Read the model definition and answer for the solid it produces. Units are mm, in the model's axes. Give positions to 0.01 mm unless a question says otherwise; leave off trailing zeros. Order: outer loops, then holes, each group sorted by start corner. A loop starts at its lowest first (then second) coordinate and runs counter-clockwise, first axis right, second up. Notation, with made-up numbers: (28.5, 83.25) - (64.5, 83.25) arc R5 cw to (64.5, 88.25) - close; hole circle Ø2 at (37.5, -38). An arc over 180 degrees is marked (long way). Return JSON: item names as keys, results as strings.
```python
from build123d import *

# Parameters (mm, degrees)
F0_R          = 11
F1_DEPTH      = 37
F3_DEPTH      = 11.001
F3_DEPTH_BACK = 11.001


with BuildPart() as f1:
    # F0 (on Top) → F1 (new body)
    with BuildSketch(Plane.XY):
        Circle(F0_R)
    extrude(amount=F1_DEPTH)

    # F2 (on Front) → F3 (cut, two sides)
    with BuildSketch(Plane.XZ) as f3_sk:
        Polygon((11, 37), (-11, 37), (-11, 34.5), align=None)
    extrude(amount=-F3_DEPTH, mode=Mode.SUBTRACT)
    extrude(f3_sk.sketch, amount=F3_DEPTH_BACK, mode=Mode.SUBTRACT)

    # F4 (on face) → F5 (revolve, cut)
    with BuildSketch(Plane(origin=(-4.010708822, 0, 35.2942376339), x_dir=(0.9936052548, 0, 0.112909688), z_dir=(-0.112909688, 0, 0.9936052548))):
        with BuildLine():
            Line((12.7865213476, 0), (-4.7134786524, 0))
            ThreePointArc((-4.7134786524, 0), (4.0365213476, -8.75), (12.7865213476, 0))
        make_face()
    revolve(axis=Axis((0, 0, 35.75), (0.9936052548, 0, 0.112909688)), mode=Mode.SUBTRACT)


solid = f1.part
```
Q1. A cutting plane is placed at B-B (z = 6). Write down the section's boundary in (x, y).
Values:
{"outline": "circle Ø22 at (0, 0)"}
Q2. Given pin 1 (12 mm diameter, centred on x = -7, z = 10.5, fed in from -Y); pin 2 (1 mm diameter, centred on x = 2, z = 19, fed in from -Y); pin 3 (4 mm diameter, centred on x = 3.5, z = 7.5, fed in from +Y), each flat-ended and moving along its own axis, determine where each tip first touches the part or whether it passes through.
Values:
{"pin 1": "stops at y = -10.95", "pin 2": "stops at y = -10.9", "pin 3": "stops at y = 10.9"}
Q3. A cutting plane is placed at D-D (z = 30). Write down the section's boundary in (x, y), and give its area (3 significant figures).
Values:
{"outline": "circle Ø22 at (0, 0); hole circle Ø13.19 at (0, 0)", "area": "243 mm²"}
Q4. A cutting plane is placed at A-A (x = 6.5). Write down the section's boundary in (y, z), and give its area (3 significant figures).
Values:
{"outline": "(-8.87, 0) - (8.87, 0) - (8.87, 36.49) - (5.81, 36.49) arc R5.86 cw (long way) to (-5.81, 36.49) - (-8.87, 36.49) - close", "area": "585 mm²"}
Q5. A cutting plane is placed at C-C (y = -7.75). Write down the section's boundary in (x, z), and give its area (3 significant figures).
Values:
{"outline": "(-7.81, 0) - (7.81, 0) - (7.81, 36.64) - (4.04, 36.21) arc R4.06 cw to (-4.04, 35.29) - (-7.81, 34.86) - close", "area": "532 mm²"}
Q6. Consider L1, parallel to Y at x = 7, z = 32; L2, parallel to Y at x = 1.5, z = 32.5; L3, parallel to X at y = -0.25, z = 13. Determine where each line is inside the solid, lowest interval first.
Values:
{"L1": "y = -8.49 to -3.67, 3.67 to 8.49", "L2": "y = -10.9 to -7.98, 7.98 to 10.9", "L3": "x = -11 to 11"}
